Input: part model. Units: mm. Frame: model coordinates. A direction names the side the tool comes from. Coordinates: 2 decimals unless noted, no trailing zeros. Loops run counter-clockwise (first coordinate to the right, second up) from the corner with the lowest first, then second, coordinate; pieces in that order, holes last.
Autodesk Inventor part; units mm, degrees
ref_plane "YZ Plane" through (0, 0, 0) normal (1, 0, 0) x (0, 1, 0)
ref_plane "XZ Plane" through (0, 0, 0) normal (0, 1, 0) x (-1, 0, 0)
ref_plane "XY Plane" through (0, 0, 0) normal (0, 0, 1) x (1, 0, 0)
sketch "Sketch1" plane through (0, 0, 0) normal (0, 0, 1) x (1, 0, 0)
  line L0 (0, 0) -> (279.4, 0)
  line L1 (279.4, 0) -> (279.4, 279.4)
  line L2 (279.4, 279.4) -> (0, 279.4)
  line L3 (0, 279.4) -> (0, 0)
  dimension "d0" = 279.4
  dimension "d1" = 279.4
extrude "Extrusion1" add sketch "Sketch1" along normal blind 25.4
sketch "Sketch2" plane through (0, 0, 25.4) normal (0, 0, 1) x (1, 0, 0)
  line L0 (0, 279.4) -> (0, 0)
  line L1 (0, 213.36) -> (266.7, 213.36)
  line L2 (266.7, 213.36) -> (266.7, 226.06)
  line L3 (266.7, 226.06) -> (0, 226.06)
  line L4 (0, 226.06) -> (0, 213.36)
  line L5 (279.4, 279.4) -> (0, 279.4)
  line L6 (0, 106.68) -> (266.7, 106.68)
  line L7 (266.7, 106.68) -> (266.7, 119.38)
  line L8 (266.7, 119.38) -> (0, 119.38)
  line L9 (0, 119.38) -> (0, 106.68)
  line L10 (0, 0) -> (266.7, 0)
  line L11 (266.7, 0) -> (266.7, 12.7)
  line L12 (266.7, 12.7) -> (0, 12.7)
  line L13 (0, 12.7) -> (0, 0)
  line L14 (0, 53.34) -> (266.7, 53.34)
  line L15 (266.7, 53.34) -> (266.7, 66.04)
  line L16 (266.7, 66.04) -> (0, 66.04)
  line L17 (0, 66.04) -> (0, 53.34)
  line L18 (0, 160.02) -> (266.7, 160.02)
  line L19 (266.7, 160.02) -> (266.7, 172.72)
  line L20 (266.7, 172.72) -> (0, 172.72)
  line L21 (0, 172.72) -> (0, 160.02)
  point P0 (0, 226.06)
  point P1 (0, 172.72)
  point P2 (0, 119.38)
  point P3 (0, 66.04)
  point P4 (0, 12.7)
  dimension "d4" = 266.7
  dimension "d5" = 12.7
  dimension "d6" = 53.34
  dimension "d7" = 266.7
  dimension "d8" = 0
  dimension "d9" = 0
  dimension "d10" = 0
  dimension "d11" = 0
  dimension "d12" = 266.7
  dimension "d13" = 266.7
  dimension "d14" = 266.7
  dimension "d15" = 12.7
  dimension "d16" = 40.64
  dimension "d17" = 12.7
  dimension "d18" = 40.64
  dimension "d19" = 12.7
  dimension "d20" = 12.7
  dimension "d21" = 40.64
  dimension "d22" = 40.64
extrude "Extrusion2" cut sketch "Sketch2" against normal blind 12.7
sketch "Sketch3" plane through (0, 0, 0) normal (-1, 0, 0) x (0, 0, 1)
  line L0 (0, 279.4) -> (0, 0)
  line L1 (12.7, 226.06) -> (25.4, 226.06)
  line L2 (0, 279.4) -> (25.4, 279.4)
  line L3 (25.4, 279.4) -> (25.4, 226.06)
  line L4 (25.4, 226.06) -> (0, 226.06)
  line L5 (0, 226.06) -> (0, 279.4)
  line L6 (25.4, 213.36) -> (12.7, 213.36)
  line L7 (25.4, 213.36) -> (0, 213.36)
  line L8 (0, 213.36) -> (0, 172.72)
  line L9 (0, 172.72) -> (25.4, 172.72)
  line L10 (25.4, 172.72) -> (25.4, 213.36)
  line L11 (25.4, 160.02) -> (25.4, 119.38)
  line L12 (25.4, 160.02) -> (0, 160.02)
  line L13 (0, 160.02) -> (0, 119.38)
  line L14 (0, 119.38) -> (25.4, 119.38)
  line L15 (25.4, 119.38) -> (25.4, 160.02)
  line L16 (25.4, 106.68) -> (25.4, 66.04)
  line L17 (25.4, 106.68) -> (0, 106.68)
  line L18 (0, 106.68) -> (0, 66.04)
  line L19 (0, 66.04) -> (25.4, 66.04)
  line L20 (25.4, 66.04) -> (25.4, 106.68)
  line L21 (25.4, 53.34) -> (12.7, 53.34)
  line L22 (25.4, 53.34) -> (0, 53.34)
  line L23 (0, 53.34) -> (0, 12.7)
  line L24 (0, 12.7) -> (25.4, 12.7)
  line L25 (25.4, 12.7) -> (25.4, 53.34)
  dimension "d25" = 40.64
  dimension "d26" = 25.4
  dimension "d27" = 40.64
  dimension "d28" = 25.4
  dimension "d29" = 40.64
  dimension "d30" = 25.4
  dimension "d31" = 40.64
extrude "Extrusion3" add sketch "Sketch3" along normal blind 25.4
properties part number "NewBackPlate"
Item 1: Line query: L1, parallel to Y at x = 55.5, z = 17.75; L2, parallel to X at y = 108, z = 16.25; L3, parallel to Z at x = 157, y = 214. Output: solid intervals per line, ascending.
Result:
L1: y = 12.7 to 53.34, 66.04 to 106.68, 119.38 to 160.02, 172.72 to 213.36, 226.06 to 279.4
L2: x = 266.7 to 279.4
L3: z = 0 to 12.7
Item 2: Section query C-C (y = 113.5). Output: boundary loops of the cut face in (x, z).
Result:
outline: (0, 0) - (279.4, 0) - (279.4, 25.4) - (266.7, 25.4) - (266.7, 12.7) - (0, 12.7) - close
Item 3: Mould query, pull axis Y, two halves, no side actions, for faces 5 (the face through (131, 113, 12.7)), 6 (the face through (129, 279.4, 13)), 7 (the face through (-25.4, 140, 13)), 8 (the face through (0, 166, 6)). Classes: +Y half, -Y half, draft (parallel to the pull), parting line (faces both ways), or undercut.
Result:
face 5: undercut
face 6: +Y half
face 7: draft
face 8: undercut
Item 4: Contact query for flat-ended pins moving along their axis: P1, Ø6.5, axis at y = 62, z = 8.5, coming from the -X side; P2, Ø6.5, axis at y = 222, z = 18.5, coming from the -X side. Output: stop coordinate, or through.
Result:
P1: stops at x = 0
P2: stops at x = 266.7
Item 5: Reachability of faces 1 (the face through (0, 220, 6)), 2 (the face through (266.7, 60, 19)), 3 (the face through (-25.4, 33, 13)), 4 (the face through (266.7, 6, 19)) from +Z, -Z, +X, -X, +Y, -Y: full face, straight path, thin tool, end or side. Return the list, or none.
Result:
face 1: +Z, -Z, -X
face 2: +Z, -X
face 3: +Z, -Z, -X, +Y, -Y
face 4: +Z, -X, -Y
Item 6: Section query A-A (x = 84.5). Output: boundary loops of the cut face in (y, z).
Result:
outline: (0, 0) - (279.4, 0) - (279.4, 25.4) - (226.06, 25.4) - (226.06, 12.7) - (213.36, 12.7) - (213.36, 25.4) - (172.72, 25.4) - (172.72, 12.7) - (160.02, 12.7) - (160.02, 25.4) - (119.38, 25.4) - (119.38, 12.7) - (106.68, 12.7) - (106.68, 25.4) - (66.04, 25.4) - (66.04, 12.7) - (53.34, 12.7) - (53.34, 25.4) - (12.7, 25.4) - (12.7, 12.7) - (0, 12.7) - close
Item 7: Section query B-B (z = 18.25). Output: boundary loops of the cut face in (x, y), then the cut area to 3 significant figures.
Result:
outline: (-25.4, 12.7) - (266.7, 12.7) - (266.7, 0) - (279.4, 0) - (279.4, 279.4) - (-25.4, 279.4) - (-25.4, 226.06) - (266.7, 226.06) - (266.7, 213.36) - (-25.4, 213.36) - (-25.4, 172.72) - (266.7, 172.72) - (266.7, 160.02) - (-25.4, 160.02) - (-25.4, 119.38) - (266.7, 119.38) - (266.7, 106.68) - (-25.4, 106.68) - (-25.4, 66.04) - (266.7, 66.04) - (266.7, 53.34) - (-25.4, 53.34) - close
area: 66,600 mm2
